```python
from build123d import *

# Parameters (mm, degrees)
SKETCH1_R           = 1.5
BOSS_EXTRUDE1_DEPTH = 2.159
CUT_EXTRUDE1_DEPTH  = 3.159


with BuildPart() as part:
    # Sketch1 → Boss-Extrude1 (new body)
    with BuildSketch(Plane.XY):
        with BuildLine():
            Line((-9.906, 12.319), (13.634725801, 12.319))
            ThreePointArc((13.634725801, 12.319), (20.100510208, 9.640784407), (22.778725801, 3.175))
            Line((22.778725801, 3.175), (22.778725801, -3.175))
            ThreePointArc((22.778725801, -3.175), (20.100510208, -9.640784407), (13.634725801, -12.319))
            Line((13.634725801, -12.319), (-9.906, -12.319))
            ThreePointArc((-9.906, -12.319), (-16.371784407, -9.640784407), (-19.05, -3.175))
            Line((-19.05, -3.175), (-19.05, 3.175))
            ThreePointArc((-19.05, 3.175), (-16.371784407, 9.640784407), (-9.906, 12.319))
        make_face()
        with Locations((-12.7, 7.874)):
            Circle(SKETCH1_R, mode=Mode.SUBTRACT)
        with Locations((-12.7, -7.874)):
            Circle(SKETCH1_R, mode=Mode.SUBTRACT)
        with Locations((17.4625, 7.874)):
            Circle(SKETCH1_R, mode=Mode.SUBTRACT)
        with Locations((17.4625, -7.874)):
            Circle(SKETCH1_R, mode=Mode.SUBTRACT)
    extrude(amount=BOSS_EXTRUDE1_DEPTH)

    # Sketch4 → Cut-Extrude1 (cut, through all)
    with BuildSketch(Plane.XY.offset(2.159)):
        with BuildLine():
            Line((-6.755, 9.144), (10.483725801, 9.144))
            ThreePointArc((10.483725801, 9.144), (11.753725801, 7.874), (10.483725801, 6.604))
            Line((10.483725801, 6.604), (-6.755, 6.604))
            ThreePointArc((-6.755, 6.604), (-8.025, 7.874), (-6.755, 9.144))
        make_face()
        with BuildLine():
            Line((-12.7, 3.894666667), (16.428725801, 3.894666667))
            ThreePointArc((16.428725801, 3.894666667), (17.698725801, 2.624666667), (16.428725801, 1.354666667))
            Line((16.428725801, 1.354666667), (-12.7, 1.354666667))
            ThreePointArc((-12.7, 1.354666667), (-13.97, 2.624666667), (-12.7, 3.894666667))
        make_face()
        with BuildLine():
            Line((-12.7, -1.354666667), (16.428725801, -1.354666667))
            ThreePointArc((16.428725801, -1.354666667), (17.698725801, -2.624666667), (16.428725801, -3.894666667))
            Line((16.428725801, -3.894666667), (-12.7, -3.894666667))
            ThreePointArc((-12.7, -3.894666667), (-13.97, -2.624666667), (-12.7, -1.354666667))
        make_face()
        with BuildLine():
            Line((-6.755, -6.604), (10.483725801, -6.604))
            ThreePointArc((10.483725801, -6.604), (11.753725801, -7.874), (10.483725801, -9.144))
            Line((10.483725801, -9.144), (-6.755, -9.144))
            ThreePointArc((-6.755, -9.144), (-8.025, -7.874), (-6.755, -6.604))
        make_face()
    extrude(amount=-CUT_EXTRUDE1_DEPTH, mode=Mode.SUBTRACT)


solid = part.part
```
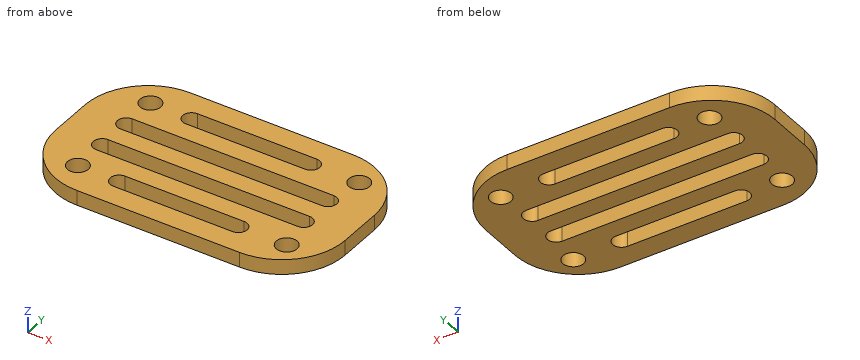
Here's how the part is built. I have some questions about the finished solid (model axes, mm). Give positions to 0.01 mm unless a question says otherwise; leave off trailing zeros. Order: outer loops, then holes, each group sorted by start corner. A loop starts at its lowest first (then second) coordinate and runs counter-clockwise, first axis right, second up. Notation, with made-up numbers: (29, 20.25) - (85, 20.25) arc R26 ccw to (85, 59.25) - close; hole circle Ø6 at (68, 3.5). An arc over 180 degrees is marked (long way). Answer as a JSON object with one key per item and string values. Group by question number.
Item 1: Please list where these lines run through material, in increasing order: probe 1 along Y at (x, z) = (-1.5, 2.05); probe 2 along Y at (x, z) = (-9.5, 0.4); probe 3 along X at (y, z) = (6.75, 0.25).
Item 2: If we section it at A-A on x = -2: Please give me the cut outline in (y, z), and give its area (3 significant figures).
Item 3: For P1, Ø4, axis at x = 5, y = -10, coming from the -Z side, with a flat end and sliding along its axis, tell me the tip position at first contact or that it passes through.
Item 4: If we section it at C-C on y = 8.75: Please give me the cut outline in (x, z).
Item 5: If we section it at B-B on z = 1.05: Give the number of separate pieces and of enclosed holes in the cut face, and give its area (3 significant figures).
Result set:
{
 "1": {"probe 1": "-12.32 to -9.14, -6.6 to -3.89, -1.35 to 1.35, 3.89 to 6.6, 9.14 to 12.32", "probe 2": "-12.32 to -3.89, -1.35 to 1.35, 3.89 to 12.32", "probe 3": "-18.32 to -13.69, -11.71 to -7.35, 11.07 to 16.47, 18.46 to 22.05"},
 "2": {"outline": "(-12.32, 0) - (-9.14, 0) - (-9.14, 2.16) - (-12.32, 2.16) - close; (-6.6, 0) - (-3.89, 0) - (-3.89, 2.16) - (-6.6, 2.16) - close; (-1.35, 0) - (1.35, 0) - (1.35, 2.16) - (-1.35, 2.16) - close; (3.89, 0) - (6.6, 0) - (6.6, 2.16) - (3.89, 2.16) - close; (9.14, 0) - (12.32, 0) - (12.32, 2.16) - (9.14, 2.16) - close", "area": "31.3 mm²"},
 "3": {"P1": "z = 0"},
 "4": {"outline": "(-17.15, 0) - (-13.92, 0) - (-13.92, 2.16) - (-17.15, 2.16) - close; (-11.48, 0) - (-7.67, 0) - (-7.67, 2.16) - (-11.48, 2.16) - close; (11.4, 0) - (16.24, 0) - (16.24, 2.16) - (11.4, 2.16) - close; (18.68, 0) - (20.88, 0) - (20.88, 2.16) - (18.68, 2.16) - close"},
 "5": {"separate pieces": "1", "enclosed holes": "8", "area": "675 mm²"}
}
